from build123d import *

# Parameters (mm, degrees)
SKETCH1_W           = 92.2
SKETCH1_H           = 170
BOX_DEPTH           = 90
SKETCH2_W           = 84.2
SKETCH2_H           = 162
BOX_CUT_DEPTH       = 86
BOSS_EXTRUDE2_DEPTH = 20
SKETCH4_W           = 24
SKETCH4_H           = 82
SKETCH4_W_2         = 45.2
SKETCH4_H_2         = 30
CUT_EXTRUDE2_DEPTH  = 4
SKETCH5_W           = 40
SKETCH5_H           = 20
CUT_EXTRUDE3_DEPTH  = 104
SKETCH6_W           = 50
SKETCH6_H           = 30
CUT_EXTRUDE4_DEPTH  = 14
SKETCH7_W           = 92.2
SKETCH7_H           = 97
CUT_EXTRUDE5_DEPTH  = 60
CUT_EXTRUDE6_DEPTH  = 100


with BuildPart() as part:
    # Sketch1 → Box (new body)
    with BuildSketch(Plane(origin=(0, 0, 0), x_dir=(1, 0, 0), z_dir=(0, 1, 0))):
        Rectangle(SKETCH1_W, SKETCH1_H)
    extrude(amount=BOX_DEPTH)

    # Sketch2 → Box Cut (cut)
    with BuildSketch(Plane(origin=(0, 90, 0), x_dir=(1, 0, 0), z_dir=(0, 1, 0))):
        Rectangle(SKETCH2_W, SKETCH2_H)
    extrude(amount=-BOX_CUT_DEPTH, mode=Mode.SUBTRACT)

    # Inside Walls → Boss-Extrude2 (add)
    with BuildSketch(Plane(origin=(0, 4, 0), x_dir=(1, 0, 0), z_dir=(0, 1, 0))):
        Polygon((-42.1, -9), (-42.1, -12), (16.1, -12), (16.1, -81), (19.1, -81), (19.1, -9), (15.9, -9), (15.9, 81), (12.9, 81), (12.9, -9), align=None)
    extrude(amount=BOSS_EXTRUDE2_DEPTH)

    # Sketch4 → Cut-Extrude2 (cut)
    with BuildSketch(Plane(origin=(0, 0, -85), x_dir=(-1, 0, 0), z_dir=(0, 0, -1))):
        with Locations((-30.1, 45)):
            Rectangle(SKETCH4_W, SKETCH4_H)
        with Locations((19.5, 19)):
            Rectangle(SKETCH4_W_2, SKETCH4_H_2)
    extrude(amount=-CUT_EXTRUDE2_DEPTH, mode=Mode.SUBTRACT)

    # Sketch5 → Cut-Extrude3 (cut)
    with BuildSketch(Plane.ZY.offset(46.1)):
        with Locations((-49.995549612, 50)):
            Rectangle(SKETCH5_W, SKETCH5_H)
    extrude(amount=-CUT_EXTRUDE3_DEPTH, mode=Mode.SUBTRACT)

    # Sketch6 → Cut-Extrude4 (cut)
    with BuildSketch(Plane.XY.offset(85)):
        with Locations((-8.9, 50)):
            Rectangle(SKETCH6_W, SKETCH6_H)
    extrude(amount=-CUT_EXTRUDE4_DEPTH, mode=Mode.SUBTRACT)

    # Sketch7 → Cut-Extrude5 (cut)
    with BuildSketch(Plane(origin=(0, 90, 0), x_dir=(1, 0, 0), z_dir=(0, 1, 0))):
        with Locations((0, 36.5)):
            Rectangle(SKETCH7_W, SKETCH7_H)
    extrude(amount=-CUT_EXTRUDE5_DEPTH, mode=Mode.SUBTRACT)

    # Sketch8 → Cut-Extrude6 (cut)
    with BuildSketch(Plane(origin=(46.1, 0, 0), x_dir=(0, 0, -1), z_dir=(1, 0, 0))):
        Polygon((-12, 30), (-47, 90), (-12, 90), align=None)
    extrude(amount=-CUT_EXTRUDE6_DEPTH, mode=Mode.SUBTRACT)


solid = part.part
Could you check a few things on this model? Use its own coordinates, in mm. A direction names the side the tool comes from. Coordinates: 2 decimals unless noted, no trailing zeros. Order: outer loops, then holes, each group sorted by start corner. A loop starts at its lowest first (then second) coordinate and runs counter-clockwise, first axis right, second up. Notation, with made-up numbers: (83.25, 89) - (131.25, 89) arc R24 ccw to (131.25, 112) - close; hole circle Ø3 at (-19.75, 26). An arc over 180 degrees is marked (long way). Answer in a Markdown table with one row per item. Add a question column.
(1) If we section it at C-C, the plane y = 14.5: Please give me the cut outline in (x, z), then the cut area to 3 significant figures.
(2) If we mould it in two halves opening along Z, with no side actions, what happens to faces 4 (the face through (16.1, 50, 83)), 5 (the face through (18, 48, 81)), 6 (the face through (7, 10, -85))? For each: released by +Z, released by -Z, zero draft, split by the parting line, or undercut.
(3) On a 3-axis mill with a long thin cutter (end or side, diameter ignored), from which of +Z, -Z, +X, -X, +Y, -Y can I reach the whole of each face in a straight line? I mean faces 1 (the face through (19.1, 14, 46)), 2 (the face through (12.9, 14, -37)), 3 (the face through (10, 30, -83)). Say none if no direction works.
(4) I need wall thicknesses on L1, parallel to X at y = 22.5, z = 15.5; L2, parallel to X at y = 48, z = 60.5; L3, parallel to Z at x = 25.5, y = 42. Which ranges of each line are inside material? Lowest first, please.
(5) Will these pins go through, and if not, where does the flat tip stop? pin 1 (13 mm diameter, centred on x = 31.5, z = -25.5, fed in from +Y); pin 2 (2 mm diameter, centred on x = 14.5, z = -47.5, fed in from +Y); pin 3 (10 mm diameter, centred on x = -4, y = 12.5, fed in from -Z).
(6) If we section it at B-B, the plane x = -27: Please give me the cut outline in (y, z), then the cut area to 3 significant figures.
(7) If we section it at D-D, the plane y = 75: Please give me the cut outline in (x, z), then the cut area to 3 significant figures.
(8) If we section it at A-A, the plane y = 28: Please give me the cut outline in (x, z).
Results are:
| question | item | result |
|---|---|---|
| 1 | outline | (-46.1, -85) - (-42.1, -85) - (-42.1, 9) - (12.9, 9) - (12.9, -81) - (3.1, -81) - (3.1, -85) - (18.1, -85) - (18.1, -81) - (15.9, -81) - (15.9, 9) - (19.1, 9) - (19.1, 81) - (42.1, 81) - (42.1, -85) - (46.1, -85) - (46.1, 85) - (-46.1, 85) - close; hole (-42.1, 12) - (16.1, 12) - (16.1, 81) - (-42.1, 81) - close |
| 1 | area | 2,420 mm2 |
| 2 | face 4 | zero draft |
| 2 | face 5 | undercut |
| 2 | face 6 | released by -Z |
| 3 | face 1 | -Z, +Y |
| 3 | face 2 | +Y |
| 3 | face 3 | -Z, +X, -X, +Y |
| 4 | L1 | x = -46.1 to -42.1, 16.1 to 19.1, 42.1 to 46.1 |
| 4 | L2 | x = -46.1 to -42.1, 42.1 to 46.1 |
| 4 | L3 | z = 81 to 85 |
| 5 | pin 1 | stops at y = 4 |
| 5 | pin 2 | stops at y = 24 |
| 5 | pin 3 | stops at z = 9 |
| 6 | outline | (0, -85) - (4, -85) - (4, 9) - (24, 9) - (24, 12) - (4, 12) - (4, 81) - (35, 81) - (35, 85) - (0, 85) - close; (65, 81) - (90, 81) - (90, 85) - (65, 85) - close |
| 6 | area | 964 mm2 |
| 7 | outline | (-46.1, 38.25) - (-42.1, 38.25) - (-42.1, 81) - (42.1, 81) - (42.1, 38.25) - (46.1, 38.25) - (46.1, 85) - (-46.1, 85) - close |
| 7 | area | 711 mm2 |
| 8 | outline | (-46.1, -85) - (-42.1, -85) - (-42.1, 81) - (42.1, 81) - (42.1, -85) - (46.1, -85) - (46.1, 85) - (-46.1, 85) - close; (3.1, -85) - (18.1, -85) - (18.1, -81) - (3.1, -81) - close |
